from build123d import *

# Parameters (mm, degrees)
F2_R     = 11.441982
F3_DEPTH = 11.844136
F4_R     = 8.253592
F5_DEPTH = 104.953468


with BuildPart() as f1:
    # F0 (on Front) → F1 (revolve)
    with BuildSketch(Plane.XZ):
        Polygon((33.57698, 56.775637), (0, 56.165144), (0, 0), (33.57698, 0), align=None)
    revolve(axis=Axis((0, 0, 28.082572), (0, 0, -1)))

    # F2 (on face) → F3 (join)
    with BuildSketch(Plane(origin=(0, 0, 0), x_dir=(1, 0, 0), z_dir=(0, 0, -1))):
        Circle(F2_R)
    extrude(amount=F3_DEPTH)

    # F4 (on face) → F5 (cut)
    with BuildSketch(Plane(origin=(0, 0, -11.844136), x_dir=(1, 0, 0), z_dir=(0, 0, -1))):
        Circle(F4_R)
    extrude(amount=-F5_DEPTH, mode=Mode.SUBTRACT)


solid = f1.part
Work out the finished part from the listing and answer in its coordinate system (mm). A direction names the side the tool comes from. Give positions to 0.01 mm unless a question says otherwise; leave off trailing zeros. Write each loop counter-clockwise with the first axis right and the second up, starting at its lowest first coordinate (ties: lowest second). Pieces come first, ordered by that corner, then holes.
Q1. Given pin 1 (10 mm diameter, centred on x = -20, y = 5, fed in from +Z); pin 2 (1.5 mm diameter, centred on x = 8.5, z = 23.5, fed in from +Y); pin 3 (10 mm diameter, centred on x = 0, y = 0, fed in from -Z); pin 4 (3 mm diameter, centred on y = -20.5, z = 12.5, fed in from +X), each flat-ended and moving along its own axis, determine where each tip first touches the part or whether it passes through.
Answer:
pin 1: stops at z = 56.63
pin 2: stops at y = 32.67
pin 3: passes through
pin 4: stops at x = 27.68
Q2. The part is cut by section C-C on z = 21.5. Give the vertices of the cut face in (x, y), and give its area (3 significant figures).
Answer:
outline: circle Ø67.15 at (0, 0); hole circle Ø16.51 at (0, 0)
area: 3,330 mm2
Q3. A tool of negligible diameter and unlimited length cuts with its end or side. For faces 4 (the face through (10.914, -3.437, -5.839)), 5 (the face through (3, 8, -11.844)), from which of +Z, -Z, +X, -X, +Y, -Y can it reach the whole face along a straight path? Write none if from no direction.
Answer:
face 4: -Z
face 5: -Z, +X, -X, +Y, -Y
Q4. For a pull along X with two mould halves and no side action, classify faces 1 (the face through (32.026, -10.086, 28.785)), 2 (the face through (9.045, -2.848, 56.338)), 3 (the face through (-14, 0, 0)) as released by +X, released by -X, zero draft, split by the parting line, or undercut.
Answer:
face 1: split by the parting line
face 2: undercut
face 3: zero draft
Q5. The part is cut by section A-A on x = 0. Give the vertices of the cut face in (y, z), and give its area (3 significant figures).
Answer:
outline: (-33.58, 0) - (-11.44, 0) - (-11.44, -11.84) - (-8.25, -11.84) - (-8.25, 56.32) - (-33.58, 56.78) - close; (8.25, -11.84) - (11.44, -11.84) - (11.44, 0) - (33.58, 0) - (33.58, 56.78) - (8.25, 56.32) - close
area: 2,940 mm2
Q6. The part is cut by section D-D on z = -5. Give the vertices of the cut face in (x, y), and give its area (3 significant figures).
Answer:
outline: circle Ø22.88 at (0, 0); hole circle Ø16.51 at (0, 0)
area: 197 mm2
Q7. Straight lines are drawn through the part: L1, parallel to Y at x = 0, z = 26.5; L2, parallel to X at y = 2, z = 50. For each, find the intervals that lie inside material, in ascending order.
Answer:
L1: y = -33.58 to -8.25, 8.25 to 33.58
L2: x = -33.52 to -8.01, 8.01 to 33.52
